Autodesk Inventor part; units mm, degrees
ref_plane "YZ Plane" through (0, 0, 0) normal (1, 0, 0) x (0, 1, 0)
ref_plane "XZ Plane" through (0, 0, 0) normal (0, 1, 0) x (-1, 0, 0)
ref_plane "XY Plane" through (0, 0, 0) normal (0, 0, 1) x (1, 0, 0)
sketch "Sketch1" plane through (0, 0, 0) normal (0, 0, 1) x (1, 0, 0)
  circle A0 centre (0, 0) radius 22.5
  arc A1 (7.2901, 17.5999) -> (-7.2901, 17.5999) centre (0, 0) ccw
  line L0 (-7.2901, 17.5999) -> (-7.5205, 17.5027)
  line L1 (-4.7835, 11.5485) -> (-4.8792, 11.7795)
  line L2 (-7.5205, 17.5027) -> (-4.7835, 11.0159)
  line L3 (-11.5485, 4.7835) -> (-11.7795, 4.8792)
  line L4 (-11.7795, 4.8792) -> (-4.8792, 11.7795)
  line L5 (0, 0) -> (-3.3576, 3.3576)
  line L6 (0, 0) -> (0, 3.3576)
  line L7 (0, 0) -> (-2.7445, 0)
  line L8 (-17.5027, 7.5205) -> (-11.0159, 4.7835)
  line L9 (0, 0) -> (2.6435, 2.6435)
  line L10 (7.5205, -17.5027) -> (4.7835, -11.0159)
  line L11 (4.8792, -11.7795) -> (11.7795, -4.8792)
  line L12 (17.5027, -7.5205) -> (11.0159, -4.7835)
  line L13 (17.5027, 7.5205) -> (11.0159, 4.7835)
  line L14 (11.7795, 4.8792) -> (4.8792, 11.7795)
  line L15 (7.5205, 17.5027) -> (4.7835, 11.0159)
  line L16 (-17.5027, -7.5205) -> (-11.0159, -4.7835)
  line L17 (-11.7795, -4.8792) -> (-4.8792, -11.7795)
  line L18 (-7.5205, -17.5027) -> (-4.7835, -11.0159)
  arc A2 (-17.5027, 7.5205) -> (-17.5027, -7.5205) centre (0, 0) ccw
  arc A3 (-7.5205, -17.5027) -> (7.5205, -17.5027) centre (0, 0) ccw
  arc A4 (17.5027, -7.5205) -> (17.5027, 7.5205) centre (0, 0) ccw
  arc A5 (7.5205, 17.5027) -> (-7.5205, 17.5027) centre (0, 0) ccw
  line L19 (17.5027, 7.5205) -> (18.4489, 7.9197)
  line L20 (7.5205, 17.5027) -> (7.9197, 18.4489)
  line L21 (-17.5027, 7.5205) -> (-18.4489, 7.9197)
  line L22 (-7.5205, 17.5027) -> (-7.9197, 18.4489)
  line L23 (17.5027, -7.5205) -> (18.4489, -7.9197)
  line L24 (7.5205, -17.5027) -> (7.9197, -18.4489)
  line L25 (-7.5205, -17.5027) -> (-7.9197, -18.4489)
  line L26 (-17.5027, -7.5205) -> (-18.4489, -7.9197)
  arc A6 (7.5496, 17.5718) -> (-7.5496, 17.5718) centre (0, 0) ccw
  arc A7 (17.5718, -7.5496) -> (17.5718, 7.5496) centre (0, 0) ccw
  arc A8 (-17.5718, 7.5496) -> (-17.5718, -7.5496) centre (0, 0) ccw
  arc A9 (-7.5496, -17.5718) -> (7.5496, -17.5718) centre (0, 0) ccw
  point P0 (-5.0385, -11.6202)
  point P1 (-11.6202, -5.0385)
  point P2 (-11.6202, 5.0385)
  point P3 (-5.0385, 11.6202)
  point P4 (5.0385, 11.6202)
  point P5 (11.6202, 5.0385)
  point P6 (11.6202, -5.0385)
  point P7 (5.0385, -11.6202)
  dimension "d0" = 45
  dimension "d1" = 0.25
  dimension "d2" = 0.25
  dimension "d3" = 0.25
extrude "Extrusion1" add sketch "Sketch1" along normal blind 20
sketch "Sketch2" plane through (0, 0, 20) normal (0, 0, 1) x (1, 0, 0)
  circle A0 centre (13.946, 0) radius 2.875
  circle A1 centre (0, -13.946) radius 2.875
  circle A2 centre (-13.946, 0) radius 2.875
  circle A3 centre (0, 13.946) radius 2.875
  point P0 (0, 0)
  point P1 (0, 0)
  dimension "d7" = 5.75
  dimension "d8" = 5.75
  dimension "d9" = 5.75
  dimension "d10" = 5.75
extrude "Extrusion2" add sketch "Sketch2" against normal blind 5
sketch "Sketch3" plane through (0, 0, 20) normal (0, 0, 1) x (1, 0, 0)
  circle A0 centre (0, 0) radius 22.5
extrude "Extrusion3" add sketch "Sketch3" along normal blind 5
sketch "Sketch4" plane through (0, 0, 25) normal (0, 0, 1) x (1, 0, 0)
  line L0 (-5, -5) -> (5, -5)
  line L1 (5, -5) -> (5, 5)
  line L2 (5, 5) -> (-5, 5)
  line L3 (-5, 5) -> (-5, -5)
  line L4 (-5, -5) -> (5, 5) construction
  line L5 (5, -5) -> (-5, 5) construction
  circle A0 centre (0, 0) radius 22.5
  line L6 (5, 5) -> (-3.5794, 5)
  line L7 (5, 5) -> (-5, 5)
  line L8 (-5, 5) -> (-5, 25)
  line L9 (-5, 25) -> (5, 25)
  line L10 (5, 25) -> (5, 5)
  line L11 (-4.9693, -4.9693) -> (-24.9693, -4.9693)
  line L12 (-24.9693, -4.9693) -> (-24.9693, 5.0307)
  line L13 (-24.9693, 5.0307) -> (-4.9693, 5.0307)
  line L14 (-4.9693, 5.0307) -> (-4.9693, -4.9693)
  line L15 (-4.9693, -4.9693) -> (5.0307, -4.9693)
  line L16 (5.0307, -4.9693) -> (5.0307, -24.9693)
  line L17 (5.0307, -24.9693) -> (-4.9693, -24.9693)
  line L18 (-4.9693, -24.9693) -> (-4.9693, -4.9693)
  line L19 (5.0307, -4.9693) -> (25.0307, -4.9693)
  line L20 (25.0307, -4.9693) -> (25.0307, 5.0307)
  line L21 (25.0307, 5.0307) -> (5.0307, 5.0307)
  line L22 (5.0307, 5.0307) -> (5.0307, -4.9693)
  circle A1 centre (0, 0) radius 22.5
  point P0 (-4.9693, -5)
  point P1 (-4.9693, -21.9444)
  point P2 (5.0307, -21.9304)
  point P3 (5, -4.9693)
  point P4 (-5, 5.0307)
  point P5 (-21.9304, 5.0307)
  point P6 (-21.9444, -4.9693)
  point P7 (-5, -4.9693)
  point P8 (5, 21.9374)
  point P9 (-5, 21.9374)
  point P10 (21.9444, -4.9693)
  point P11 (21.9304, 5.0307)
  dimension "d15" = 10
  dimension "d16" = 10
  dimension "d17" = 10
  dimension "d18" = 20
  dimension "d19" = 20
  dimension "d20" = 10
  dimension "d21" = 10
  dimension "d22" = 20
  dimension "d23" = 20
  dimension "d24" = 10
extrude "Extrusion4" add sketch "Sketch4" along normal blind 25 contours L0 L1 L15 L16 A0 L18 | L11 A0 L13 L8 L3 | L14 L2 L1 L15 | L14 L13 L8 A0 L10 L2 | L22 L21 A0 L19
properties part number "3xxx_Tx_Coil_Winding_MPSv2_v1.form"
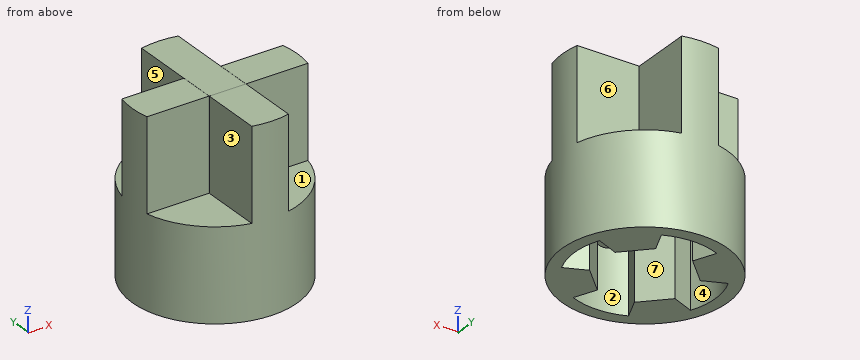
Here's how the part is built. I have some questions about the finished solid (model axes, mm). Face numbers are marked on the shaded views. A direction names the side the tool comes from. Give positions to 0.01 mm unless a question says otherwise; leave off trailing zeros. Write each loop counter-clockwise with the first axis right and the second up, starting at its lowest first coordinate (ties: lowest second). Pieces come first, ordered by that corner, then holes. Notation, with made-up numbers: M 2,-32.75 L 60,-32.75 A14 ccw 60,-9.75 Z; hole C -15,-18 d4. An arc over 180 degrees is marked long. Put each result on its own line as item: value. Start each with the question number.
Item 1: If we section it at C-C, the plane z = 9.5: Write out the boundary of the cut face in (x, y).
Item 2: If we section it at D-D, the plane x = -10: Write out the boundary of the cut face in (y, z).
Item 3: Will these pins go through, and if not, where does the flat tip stop? pin 1 (8 mm diameter, centred on y = -5.5, z = 13, fed in from +X); pin 2 (1.7 mm diameter, centred on x = -1.5, y = 14.5, fed in from -Z); pin 3 (12 mm diameter, centred on x = -3, z = 40.5, fed in from -Y).
Item 4: Thinking about a two-plate mould opening in X: for the marked faces 4, 5, 6 and 7, which applies, +X half, -X half, draft (parallel to the pull), parting line (faces both ways), or undercut?
Item 5: On a 3-axis mill with a long thin cutter (end or side, diameter ignored), from which of +Z, -Z, +X, -X, +Y, -Y can I reach the whole of each face in a straight line? I mean the marked faces 1, 2 and 3. Say none if no direction works.
Item 6: I need wall thicknesses on L1, parallel to Y at x = -0.5, z = 6; L2, parallel to X at y = 5.5, z = 6; L3, parallel to X at y = 16.5, z = 16.5. Which ranges of each line are inside material? Lowest first, please. Write a range as from..to.
Values:
1. outline: C 0,0 d45; hole M -17.57,-7.55 L -17.5,-7.52 L -11.62,-5.04 L -5.04,-11.62 L -7.52,-17.5 L -7.55,-17.57 A19.12 ccw 7.55,-17.57 L 7.52,-17.5 L 5.04,-11.62 L 11.62,-5.04 L 17.5,-7.52 L 17.57,-7.55 A19.12 ccw 17.57,7.55 L 17.5,7.52 L 11.62,5.04 L 5.04,11.62 L 7.52,17.5 L 7.55,17.57 A19.12 ccw -7.55,17.57 L -7.52,17.5 L -5.04,11.62 L -11.62,5.04 L -17.5,7.52 L -17.57,7.55 A19.12 ccw Z
2. outline: M -20.16,0 L -6.66,0 L -6.66,20 L 6.66,20 L 6.66,0 L 20.16,0 L 20.16,25 L 5.03,25 L 5.03,50 L -4.97,50 L -4.97,25 L -20.16,25 Z
3. pin 1: x = 22.45
3. pin 2: z = 15
3. pin 3: y = -22.5
4. face 4: undercut
4. face 5: -X half
4. face 6: draft
4. face 7: undercut
5. face 1: +Z, +X, -Y
5. face 2: -Z
5. face 3: +Z, -X, -Y
6. L1: -22.49..-19.12, 19.12..22.49
6. L2: -21.82..-18.32, -12.71..-11.16, 11.16..12.71, 18.32..21.82
6. L3: -15.3..-7.1, -1.32..1.32, 7.1..15.3
